CAD build for the part. Positions are in the model's coordinates, mm. A direction names the side the tool comes from. Give positions to 0.01 mm unless a question says otherwise; leave off trailing zeros. Write each loop counter-clockwise with the first axis right and the second up, starting at its lowest first coordinate (ties: lowest second). Pieces come first, ordered by that corner, then holes. Notation, with made-up numbers: M -29,12 L 26,12 A21 ccw 26,39 Z; hole C 9.25,59 d9. An arc over 180 degrees is marked long. One line per question, with ' | ' between items. Start each with the question number.
1. Cut at D-D, the plane y = -9.25. Write the cut outline in (x, z).
2. Cut at B-B, the plane y = 0. Write the cut outline in (x, z) (1 decimal), then the cut area to 3 significant figures.
3. Cut at C-C, the plane z = 0. Write the cut outline in (x, y).
4. Flat gauge pins, fed straight in: pin 1 (12.5 mm diameter, centred on x = 4, y = -2.5, fed in from +Z); pin 2 (1.5 mm diameter, centred on x = -9, y = -4, fed in from +Z); pin 3 (11 mm diameter, centred on y = 0, z = 0, fed in from +X); pin 4 (10 mm diameter, centred on x = -8, y = -6, fed in from -Z). Where does each tip first touch, or does it go through?
5. Pull direction Z, two halves, no side cores. Call faces 3 (the face through (2.5, -2.5, 36.83)), 4 (the face through (0, 12.7, 0)): released by +Z, released by -Z, zero draft, split by the parting line, or undercut.
6. Which spindle directions (+Z, -Z, +X, -X, +Y, -Y) get a long thin tool onto all of the face, cutting with end or side? Do faces 1 (the face through (-12.7, 3, -5.5)), 2 (the face through (2.8, -1.5, -24.9)). Say none if no direction does.
7. Wall check: L1, parallel to Y at x = 6.25, z = 0; L2, parallel to X at y = 0, z = -18 (3 decimals); L3, parallel to Y at x = 5.75, z = -3. Give the ranges that are in metal, low to high.
8. Cut at A-A, the plane x = 0. Write the cut outline in (y, z) (1 decimal), then the cut area to 3 significant figures.
```python
from build123d import *

# Parameters (mm, degrees)
SKETCH1_W           = 25.4
SKETCH1_H           = 25.4
SKETCH1_R           = 4.7625
BOSS_EXTRUDE1_DEPTH = 12.7
SKETCH1_4_W         = 24.13
SKETCH1_4_H         = 3.175
SKETCH1_5_W         = 24.13
SKETCH1_5_H         = 3.175
CHAMFER1_SIZE       = 1.27


with BuildPart() as part:
    # Sketch1 → Boss-Extrude1 (new, symmetric)
    with BuildSketch(Plane(origin=(0, 0, 0), x_dir=(0, 0, -1), z_dir=(1, 0, 0))):
        Rectangle(SKETCH1_W, SKETCH1_H)
        Circle(SKETCH1_R, mode=Mode.SUBTRACT)
    extrude(amount=BOSS_EXTRUDE1_DEPTH, both=True)

    # Sketch1_4 → Revolve1 (revolve)
    with BuildSketch(Plane(origin=(0, 0, 0), x_dir=(0, 0, -1), z_dir=(1, 0, 0))):
        with Locations((-24.765, 1.5875)):
            Rectangle(SKETCH1_4_W, SKETCH1_4_H)
        with BuildLine():
            Line((-42.542324878, 0), (-36.83, 0))
            Line((-36.83, 0), (-36.83, 3.175))
            Line((-36.83, 3.175), (-36.83, 5.712324878))
            ThreePointArc((-36.83, 5.712324878), (-40.869223658, 4.039223658), (-42.542324878, 0))
        make_face()
    revolve(axis=Axis((0, 0, 12.7), (0, 0, 1)))

    # Sketch1_5 → Revolve2 (revolve)
    with BuildSketch(Plane(origin=(0, 0, 0), x_dir=(0, 0, -1), z_dir=(1, 0, 0)), mode=Mode.PRIVATE) as revolve2_sk:
        with Locations((24.765, 1.5875)):
            Rectangle(SKETCH1_5_W, SKETCH1_5_H)
        with BuildLine():
            Line((36.83, 3.175), (36.83, 0))
            Line((36.83, 0), (42.542324878, 0))
            ThreePointArc((42.542324878, 0), (40.869223658, 4.039223658), (36.83, 5.712324878))
            Line((36.83, 5.712324878), (36.83, 3.175))
        make_face()
    revolve(revolve2_sk.sketch.rotate(Axis((0, 0, -12.7), (0, 0, -1)), 180), axis=Axis((0, 0, -12.7), (0, 0, -1)))

    # Chamfer1
    chamfer1_edges = [part.edges().sort_by_distance(p)[0] for p in [
        (12.7, 0, 4.7625),
        (-12.7, 0, 4.7625),
    ]]
    chamfer(chamfer1_edges, length=CHAMFER1_SIZE)


solid = part.part
```
Here are the results:
1) outline: M -12.7,-12.7 L 12.7,-12.7 L 12.7,12.7 L -12.7,12.7 Z
2) outline: M -12.7,-12.7 L -3.2,-12.7 L -3.2,-36.8 L -5.7,-36.8 A5.7 ccw 5.7,-36.8 L 3.2,-36.8 L 3.2,-12.7 L 12.7,-12.7 L 12.7,-6 L 11.4,-4.8 L -11.4,-4.8 L -12.7,-6 Z; M -12.7,6 L -11.4,4.8 L 11.4,4.8 L 12.7,6 L 12.7,12.7 L 3.2,12.7 L 3.2,36.8 L 5.7,36.8 A5.7 ccw -5.7,36.8 L -3.2,36.8 L -3.2,12.7 L -12.7,12.7 Z | area: 809 mm^2
3) outline: M -12.7,-12.7 L 12.7,-12.7 L 12.7,-6.03 L 11.43,-4.76 L -11.43,-4.76 L -12.7,-6.03 Z; M -12.7,6.03 L -11.43,4.76 L 11.43,4.76 L 12.7,6.03 L 12.7,12.7 L -12.7,12.7 Z
4) pin 1: z = 42.54 | pin 2: z = 12.7 | pin 3: x = 12.17 | pin 4: z = -39.59
5) face 3: undercut | face 4: zero draft
6) face 1: +Z, -Z, -X, +Y, -Y | face 2: none
7) L1: -12.7 to -4.76, 4.76 to 12.7 | L2: -3.175 to 3.175 | L3: -12.7 to -3.7, 3.7 to 12.7
8) outline: M -12.7,-12.7 L -3.2,-12.7 L -3.2,-36.8 L -5.7,-36.8 A5.7 ccw 5.7,-36.8 L 3.2,-36.8 L 3.2,-12.7 L 12.7,-12.7 L 12.7,12.7 L 3.2,12.7 L 3.2,36.8 L 5.7,36.8 A5.7 ccw -5.7,36.8 L -3.2,36.8 L -3.2,12.7 L -12.7,12.7 Z; hole C 0,0 d9.5 | area: 983 mm^2
